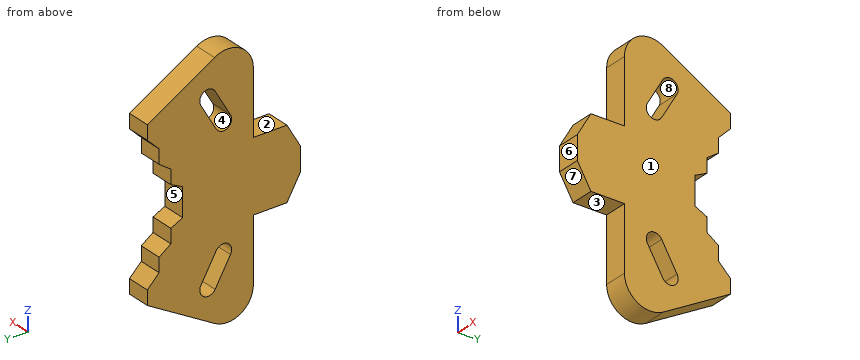
```python
from build123d import *

# Parameters (mm, degrees)
EXTRUDE_1_DEPTH = 10
SKETCH_2_W      = 30
SKETCH_2_H      = 20
EXTRUDE_2_DEPTH = 10
CHAMFER_1_SIZE  = 10
CHAMFER_1_SIZE2 = 5.773502692
CHAMFER_2_SIZE  = 10
CHAMFER_2_SIZE2 = 5.773502692


with BuildPart() as part:
    # Эскиз1 → Бобышка-Вытянуть1 (new body)
    with BuildSketch(Plane(origin=(0, 0, 0), x_dir=(0, 0, -1), z_dir=(1, 0, 0))):
        with BuildLine():
            Line((0, 0), (41.867903864, 0))
            ThreePointArc((41.867903864, 0), (51.394183306, 5.5), (51.394183306, 16.5))
            Line((51.394183306, 16.5), (34.939700634, 45))
            Line((34.939700634, 45), (28.939700634, 45))
            Line((28.939700634, 45), (23.939700634, 40))
            Line((23.939700634, 40), (17.939700634, 40))
            Line((17.939700634, 40), (14.438662943, 35))
            Line((14.438662943, 35), (8.438662943, 35))
            Line((8.438662943, 35), (6, 30))
            Line((6, 30), (0, 30))
            Line((0, 30), (0, 0))
        make_face()
        with BuildLine():
            Line((23.519083625, 15.781088913), (34.777413874, 22.281088913))
            ThreePointArc((34.777413874, 22.281088913), (39.558502787, 21), (38.277413874, 16.218911087))
            Line((38.277413874, 16.218911087), (27.019083625, 9.718911087))
            ThreePointArc((27.019083625, 9.718911087), (22.237994712, 11), (23.519083625, 15.781088913))
        make_face(mode=Mode.SUBTRACT)
    extrude(amount=EXTRUDE_1_DEPTH)

    # Зеркальное отражение1: part across plane


with BuildPart() as part_1:
    add(part.part)
    add(part.part.mirror(Plane(origin=(10, 30, 0), x_dir=(1, 0, 0), z_dir=(0, 0, -1))))

    # Эскиз2 → Бобышка-Вытянуть2 (add)
    with BuildSketch(Plane(origin=(10, 0, 0), x_dir=(0, 0, -1), z_dir=(1, 0, 0))):
        with Locations((0, -10)):
            Rectangle(SKETCH_2_W, SKETCH_2_H)
    extrude(amount=-EXTRUDE_2_DEPTH)

    # Фаска1
    chamfer_1_edges = [part_1.edges().sort_by_distance(p)[0] for p in [
        (5, -20, 15),
    ]]
    chamfer_1_side = [part_1.faces().sort_by_distance(p)[0] for p in [
        (5, -20, 0),
    ]]
    chamfer(chamfer_1_edges, length=CHAMFER_1_SIZE, length2=CHAMFER_1_SIZE2, reference=chamfer_1_side[0])

    # Фаска2
    chamfer_2_edges = [part_1.edges().sort_by_distance(p)[0] for p in [
        (5, -20, -15),
    ]]
    chamfer_2_side = [part_1.faces().sort_by_distance(p)[0] for p in [
        (5, -20, -5),
    ]]
    chamfer(chamfer_2_edges, length=CHAMFER_2_SIZE, length2=CHAMFER_2_SIZE2, reference=chamfer_2_side[0])


solid = part_1.part
```
Verification items for the finished model (mm, model axes). Face numbers are marked on the shaded views. A direction names the side the tool comes from. Give positions to 0.01 mm unless a question says otherwise; leave off trailing zeros. Loops run counter-clockwise (first coordinate to the right, second up) from the corner with the lowest first, then second, coordinate; pieces in that order, holes last. Notation, with made-up numbers: M -40,18 L -5,18 A27 cw -5,49 Z; hole C -28.5,67.5 d6. An arc over 180 degrees is marked long. Return JSON: item names as keys, results as strings.
1) Material ranges on L1, parallel to Z at x = 2.5, y = 10; L2, parallel to Y at x = 8.75, z = -21; L3, parallel to Y at x = 6, z = -35.5, recorded low to high. Write a range as [from, to].
Findings:
{"L1": "z = [-52.82, -27.51], [-23.1, 23.1], [27.51, 52.82]", "L2": "y = [0, 40]", "L3": "y = [0, 14.62], [22.6, 44.03]"}
2) Tool access check on the marked faces 1, 2, 3, 4 and 5. Record the directions out of +Z, -Z, +X, -X, +Y, -Y that give a thin tool (end or side, any length) a straight path to the whole face; none if there is none.
Findings:
{"face 1": "+Z, -Z, +X, +Y, -Y", "face 2": "+Z, +X, -X, -Y", "face 3": "-Z, +X, -X, -Y", "face 4": "+X, -X", "face 5": "+X, -X, +Y"}
3) Section check C-C, the plane y = 19.25. Enter the section's corners in (x, z), and give its area (3 significant figures).
Findings:
{"outline": "M 0,-49.81 L 10,-49.81 L 10,-40.03 L 0,-40.03 Z; M 0,-29.53 L 10,-29.53 L 10,29.53 L 0,29.53 Z; M 0,40.03 L 10,40.03 L 10,49.81 L 0,49.81 Z", "area": "786 mm2"}
4) Section check A-A, the plane x = 8.5. Count the separate pieces of the cut face and the enclosed holes in it, and give its area (3 significant figures).
Findings:
{"separate pieces": "1", "enclosed holes": "2", "area": "3,930 mm2"}
5) Mould release check, pull along Z, two halves, no side actions. Record for the marked faces 6, 7 and 8: released by +Z, released by -Z, zero draft, split by the parting line, or undercut.
Findings:
{"face 6": "zero draft", "face 7": "released by -Z", "face 8": "undercut"}
6) Section check D-D, the plane y = 27.5. Enter the section's corners in (x, z), and give its area (3 significant figures).
Findings:
{"outline": "M 0,-45.04 L 10,-45.04 L 10,45.04 L 0,45.04 Z", "area": "901 mm2"}
7) Gauge pin test, flat ends, axial feed: P1, Ø1, axis at x = 2.5, y = 17.5, coming from the +Z side; P2, Ø6, axis at x = 4.5, y = 1, coming from the +Z side; P3, Ø2, axis at x = 7.5, y = -5, coming from the -Z side. Record the tip position at first contact, or that the pin passes through.
Findings:
{"P1": "stops at z = 51.11", "P2": "stops at z = 50.35", "P3": "stops at z = -15"}
8) Section check B-B, the plane y = 12.75. Enter the section's corners in (x, z), and give its area (3 significant figures).
Findings:
{"outline": "M 0,-52.73 L 10,-52.73 L 10,-32.27 L 0,-32.27 Z; M 0,-21.77 L 10,-21.77 L 10,21.77 L 0,21.77 Z; M 0,32.27 L 10,32.27 L 10,52.73 L 0,52.73 Z", "area": "845 mm2"}
